For this review, take the finished solid that the model builds, in its own axes (mm). A direction names the side the tool comes from. Coordinates: 2 decimals unless noted, no trailing zeros. Loops run counter-clockwise (first coordinate to the right, second up) from the corner with the lowest first, then second, coordinate; pieces in that order, holes last. Notation, with made-up numbers: (48.25, -40) -> (65.25, -40) arc R20 ccw to (65.25, -13) -> close; hole circle Ø11 at (-32, 43). An arc over 180 degrees is marked (long way). Answer in a Markdown table with one row per item.
from build123d import *

# Parameters (mm, degrees)
BOSS_EXTRUDE1_START = -25.4
SKETCH2_R           = 1.905
BOSS_EXTRUDE1_DEPTH = 25.4
FILLET1_R           = 2.54


with BuildPart() as part:
    # Sketch1 → Revolve1 (revolve)
    with BuildSketch(Plane.XY):
        Polygon((-20.0787, -6.858779284), (-20.0787, 20.444981856), (-21.1836, 24.568524793), (-21.1836, 94.741220716), (-22.225, 94.741220716), (-22.225, 18.541220716), (-21.1201, 18.541220716), (-21.1201, -6.858779284), align=None)
    revolve(axis=Axis((0, 0, 0), (0, 1, 0)))

    # Sketch2 → Boss-Extrude1 (add)
    with BuildSketch(Plane(origin=(0, 94.741220716, 0), x_dir=(1, 0, 0), z_dir=(0, 1, 0)).offset(BOSS_EXTRUDE1_START)):
        with BuildLine():
            Line((25.1714, 2.9464), (22.02883002, 2.9464))
            ThreePointArc((22.02883002, 2.9464), (22.225, 0), (22.02883002, -2.9464))
            Line((22.02883002, -2.9464), (25.1714, -2.9464))
            ThreePointArc((25.1714, -2.9464), (28.1178, 0), (25.1714, 2.9464))
        make_face()
        with Locations((25.1714, 0)):
            Circle(SKETCH2_R, mode=Mode.SUBTRACT)
    extrude(amount=-BOSS_EXTRUDE1_DEPTH)

    # Fillet1
    fillet1_edges = [part.edges().sort_by_distance(p)[0] for p in [
        (22.02883002, 56.641220716, 2.9464),
        (22.02883002, 56.641220716, -2.9464),
    ]]
    fillet(fillet1_edges, radius=FILLET1_R)

    # Sketch3 → Cut-Revolve2 (revolve, cut)
    with BuildSketch(Plane.XY):
        Polygon((22.225, 69.341220716), (28.1178, 59.134591717), (28.1178, 69.341220716), align=None)
        Polygon((22.225, 43.941220716), (28.1178, 54.147849715), (28.1178, 43.941220716), align=None)
    revolve(axis=Axis((0, 0, 0), (0, -1, 0)), mode=Mode.SUBTRACT)


solid = part.part
Item 1: Take a section at C-C, the plane y = 34. State the section outline as (x, z) points (3 decimals).
Worked answers:
| item | result |
|---|---|
| outline | circle Ø44.45 at (0, 0); hole circle Ø42.367 at (0, 0) |
Item 2: Take a section at A-A, the plane x = 0. State the section outline as (y, z) points (3 decimals).
Worked answers:
| item | result |
|---|---|
| outline | (-6.859, -21.12) -> (18.541, -21.12) -> (18.541, -22.225) -> (94.741, -22.225) -> (94.741, -21.184) -> (24.569, -21.184) -> (20.445, -20.079) -> (-6.859, -20.079) -> close; (-6.859, 20.079) -> (20.445, 20.079) -> (24.569, 21.184) -> (94.741, 21.184) -> (94.741, 22.225) -> (18.541, 22.225) -> (18.541, 21.12) -> (-6.859, 21.12) -> close |
Item 3: For L1, parallel to Z at x = 1, y = 25; L2, parallel to Z at x = 0, y = 3; L3, parallel to X at y = 58.5, z = 13.5, list the stretches that pass through material, from the lowest coordinate up.
Worked answers:
| item | result |
|---|---|
| L1 | -22.2 to -21.16, 21.16 to 22.2 |
| L2 | -21.12 to -20.08, 20.08 to 21.12 |
| L3 | -17.66 to -16.32, 16.32 to 17.66 |
Item 4: For faces 4 (the cylindrical face through (4.59, 60.15, -20.68)), 5 (the cylindrical face through (16.76, 5.66, -12.85)), 6 (the flat face through (20, 94.741, -8)), list the 3-axis set-ups (+Z, -Z, +X, -X, +Y, -Y) from which the entire face can be reached by the end or side of a thin tool; tool diameter is ignored.
Worked answers:
| item | result |
|---|---|
| face 4 | +Y |
| face 5 | -Y |
| face 6 | +Z, -Z, +X, -X, +Y |
Item 5: Insertion check: pin 1 (13.5 mm diameter, centred on x = -3, z = -9, fed in from -Y); pin 2 (1.1 mm diameter, centred on x = 25, y = 60, fed in from -Z); pin 3 (2 mm diameter, centred on y = 31, z = 5, fed in from -X); pin 4 (6 mm diameter, centred on x = 25.17, z = 0, fed in from +Y). Each pin has a flat end and moves straight along its axis. Give the tip position at first contact, or say it passes through.
Worked answers:
| item | result |
|---|---|
| pin 1 | through |
| pin 2 | z = -2.95 |
| pin 3 | x = -21.86 |
| pin 4 | y = 94.74 |
Item 6: The part is to be moulded in two halves that separate along X. For faces 1 (the flat face through (-20, 18.541, -8)), 2 (the conical face through (23.825, 46.801, 1.554)), 3 (the cylindrical face through (23.27, 56.79, -0.08)), say which applies: +X half, -X half, draft (parallel to the pull), parting line (faces both ways), or undercut.
Worked answers:
| item | result |
|---|---|
| face 1 | draft |
| face 2 | +X half |
| face 3 | undercut |
Item 7: Take a section at B-B, the plane z = 0. State the section outline as (x, y) points (3 decimals).
Worked answers:
| item | result |
|---|---|
| outline | (-22.225, 18.541) -> (-21.12, 18.541) -> (-21.12, -6.859) -> (-20.079, -6.859) -> (-20.079, 20.445) -> (-21.184, 24.569) -> (-21.184, 94.741) -> (-22.225, 94.741) -> close; (20.079, -6.859) -> (21.12, -6.859) -> (21.12, 18.541) -> (22.225, 18.541) -> (22.225, 43.941) -> (23.266, 45.745) -> (23.266, 67.537) -> (22.225, 69.341) -> (22.225, 94.741) -> (21.184, 94.741) -> (21.184, 24.569) -> (20.079, 20.445) -> close; (27.076, 52.344) -> (28.118, 54.148) -> (28.118, 59.135) -> (27.076, 60.938) -> close |
